Check sheet for the modelled part. Datum: model origin and axes. Units: mm. A direction names the side the tool comes from. Give positions to 0.01 mm unless a question says otherwise; leave off trailing zeros. Loops run counter-clockwise (first coordinate to the right, second up) from the corner with the lowest first, then second, coordinate; pieces in that order, holes last. Notation, with made-up numbers: M -2,-32.5 L 35,-32.5 A14 cw 35,-26.5 Z; hole C 62,-15 d5. An arc over 180 degrees is marked long. One line per question, with ' | ' between items. Start each with the question number.
from build123d import *

# Parameters (mm, degrees)
SKETCH_1_W          = 56.52
SKETCH_1_H          = 62.3
SKETCH_1_R          = 1.7
EXTRUDE_1_DEPTH     = 2
SKETCH_2_W          = 16
SKETCH_2_H          = 16
EXTRUDE_2_DEPTH     = 2
SKETCH_3_W          = 33
SKETCH_3_H          = 8
EXTRUDE_3_DEPTH     = 8
SKETCH_4_W          = 31
SKETCH_4_H          = 6
CUT_EXTRUDE_1_DEPTH = 8
SKETCH_5_W          = 7
SKETCH_5_H          = 10
EXTRUDE_4_DEPTH     = 4


with BuildPart() as part:
    # 草图1 → 凸台-拉伸1 (new body)
    with BuildSketch(Plane(origin=(0, 0, 0), x_dir=(1, 0, 0), z_dir=(0, 1, 0))):
        Rectangle(SKETCH_1_W, SKETCH_1_H)
        with Locations(Location((25, 28.25, 0), (0, 0, 270))):
            Circle(SKETCH_1_R, mode=Mode.SUBTRACT)
        with Locations(Location((25, -28.25, 0), (0, 0, 90))):
            Circle(SKETCH_1_R, mode=Mode.SUBTRACT)
        with Locations(Location((-25, -28.25, 0), (0, 0, 270))):
            Circle(SKETCH_1_R, mode=Mode.SUBTRACT)
        with Locations(Location((-25, 28.25, 0), (0, 0, 90))):
            Circle(SKETCH_1_R, mode=Mode.SUBTRACT)
    extrude(amount=EXTRUDE_1_DEPTH)

    # 草图2 → 凸台-拉伸2 (add)
    with BuildSketch(Plane(origin=(0, 2, 0), x_dir=(1, 0, 0), z_dir=(0, 1, 0))):
        Rectangle(SKETCH_2_W, SKETCH_2_H)
    extrude(amount=EXTRUDE_2_DEPTH)

    # 草图3 → 凸台-拉伸3 (add)
    with BuildSketch(Plane(origin=(0, 2, 0), x_dir=(1, 0, 0), z_dir=(0, 1, 0))):
        with Locations((0, 26.65)):
            Rectangle(SKETCH_3_W, SKETCH_3_H)
    extrude(amount=EXTRUDE_3_DEPTH)

    # 草图4 → 切除-拉伸1 (cut)
    with BuildSketch(Plane(origin=(0, 10, 0), x_dir=(1, 0, 0), z_dir=(0, 1, 0))):
        with Locations((0, 26.65)):
            Rectangle(SKETCH_4_W, SKETCH_4_H)
    extrude(amount=-CUT_EXTRUDE_1_DEPTH, mode=Mode.SUBTRACT)

    # 草图5 → 凸台-拉伸4 (add)
    with BuildSketch(Plane(origin=(0, 2, 0), x_dir=(1, 0, 0), z_dir=(0, 1, 0))):
        with Locations((-11.76, -27.15)):
            Rectangle(SKETCH_5_W, SKETCH_5_H)
    extrude(amount=EXTRUDE_4_DEPTH)


solid = part.part
Q1. Cross-section at A-A (x = 25). Record the cut outline in (y, z).
Q2. Access from +Z, -Z, +X, -X, +Y, -Y to the whole of each face (thin tool, end or side, straight path). Record for faces 1 (the flat face through (16.5, 6, -27)), 2 (the flat face through (-8.26, 4, 27)), 3 (the flat face through (0, 6, -22.65)).
Q3. Cross-section at B-B (z = -28.25). Record the cut outline in (x, y), and give its area (3 significant figures).
Q4. Depth check by flat-ended pin: P1, Ø1.6, axis at x = 11.5, y = 1, coming from the +Z side; P2, Ø2.5, axis at x = 0.5, y = 6.5, coming from the -Z side; P3, Ø5, axis at y = 8, z = -26, coming from the -X side. Enter the tip coordinate at first touch or a pass-through.
Q5. Draft check along X on faces 4 (the flat face through (0, 3, -8)), 5 (the cylindrical face through (-25.51, 0.99, -29.87)), 6 (the flat face through (-16.5, 6, -27)). Enter one of: released by +X, released by -X, zero draft, split by the parting line, or undercut.
Q6. Material ranges on probe 1 along X at (y, z) = (0.7, 28.25); probe 2 along Z at (x, y) = (-10, 3); probe 3 along Z at (x, y) = (-3.5, 8), recorded low to high. Write a range as from..to.
Q7. Cross-section at D-D (z = 1). Record the cut outline in (x, y).
Q8. Cross-section at C-C (y = 8.25). Record the cut outline in (x, z).
Solved:
1) outline: M 0,-31.15 L 2,-31.15 L 2,-29.95 L 0,-29.95 Z; M 0,-26.55 L 2,-26.55 L 2,26.55 L 0,26.55 Z; M 0,29.95 L 2,29.95 L 2,31.15 L 0,31.15 Z
2) face 1: +Z, -Z, +X, +Y | face 2: +Z, +X, +Y | face 3: +X, -X, +Y
3) outline: M -28.26,0 L -26.7,0 L -26.7,2 L -28.26,2 Z; M -23.3,0 L 23.3,0 L 23.3,2 L 16.5,2 L 16.5,10 L 15.5,10 L 15.5,2 L -15.5,2 L -15.5,10 L -16.5,10 L -16.5,2 L -23.3,2 Z; M 26.7,0 L 28.26,0 L 28.26,2 L 26.7,2 Z | area: 115 mm²
4) P1: stops at z = 31.15 | P2: stops at z = -30.65 | P3: stops at x = -16.5
5) face 4: zero draft | face 5: undercut | face 6: released by -X
6) probe 1: x = -28.26..-26.7, -23.3..23.3, 26.7..28.26 | probe 2: z = -30.65..-29.65, -23.65..-22.65, 22.15..32.15 | probe 3: z = -30.65..-29.65, -23.65..-22.65
7) outline: M -28.26,0 L 28.26,0 L 28.26,2 L 8,2 L 8,4 L -8,4 L -8,2 L -28.26,2 Z
8) outline: M -16.5,-30.65 L 16.5,-30.65 L 16.5,-22.65 L -16.5,-22.65 Z; hole M -15.5,-29.65 L 15.5,-29.65 L 15.5,-23.65 L -15.5,-23.65 Z
